Build history of the part. All positions in model axes, mm. A direction names the side the tool comes from. Coordinates: 2 decimals unless noted, no trailing zeros. Write each loop counter-clockwise with the first axis right and the second up, starting at its lowest first coordinate (ties: lowest second). Pieces come first, ordered by that corner, then holes.
from build123d import *

# Parameters (mm, degrees)
SKETCH1_R           = 4.5
SKETCH1_R_2         = 2.5
BOSS_EXTRUDE1_DEPTH = 3.6
SKETCH2_R           = 0.75
SKETCH2_R_2         = 6.25
SKETCH2_R_3         = 4.5
SKETCH2_R_4         = 2.5
SKETCH2_R_5         = 1.5
BOSS_EXTRUDE2_DEPTH = 2.7
SKETCH3_W           = 3
SKETCH3_H           = 0.5
SKETCH3_W_2         = 0.5
SKETCH3_H_2         = 3
BOSS_EXTRUDE3_DEPTH = 0.5


with BuildPart() as part:
    # Sketch1 → Boss-Extrude1 (new body)
    with BuildSketch(Plane(origin=(0, 0, 0), x_dir=(1, 0, 0), z_dir=(0, 1, 0))):
        with Locations(Location((0, 0, 0), (0, 0, 270))):
            Circle(SKETCH1_R)
        with Locations(Location((0, 0, 0), (0, 0, 270))):
            Circle(SKETCH1_R_2, mode=Mode.SUBTRACT)
    extrude(amount=BOSS_EXTRUDE1_DEPTH)

    # Sketch2 → Boss-Extrude2 (add)
    # profile 1 of 7: a face of its own
    with BuildSketch(Plane(origin=(0, 3.6, 0), x_dir=(1, 0, 0), z_dir=(0, 1, 0))):
        with BuildLine():
            ThreePointArc((4.419417382, -4.419417382), (0, -6.25), (-4.419417382, -4.419417382))
            Line((-4.419417382, -4.419417382), (-2, -16))
            ThreePointArc((-2, -16), (0, -18.265564437), (2, -16))
            Line((2, -16), (4.419417382, -4.419417382))
        make_face()
        with Locations(Location((0, -16.25, 0), (0, 0, 90))):
            Circle(SKETCH2_R, mode=Mode.SUBTRACT)
        with Locations(Location((0, -13.25, 0), (0, 0, 90))):
            Circle(SKETCH2_R, mode=Mode.SUBTRACT)
        with Locations(Location((0, -10.25, 0), (0, 0, 90))):
            Circle(SKETCH2_R, mode=Mode.SUBTRACT)
        with Locations(Location((0, -7.25, 0), (0, 0, 90))):
            Circle(SKETCH2_R, mode=Mode.SUBTRACT)
    # profile 2 of 7: a face of its own
    with BuildSketch(Plane(origin=(0, 3.6, 0), x_dir=(1, 0, 0), z_dir=(0, 1, 0))):
        with BuildLine():
            ThreePointArc((-4.419417382, -4.419417382), (-6.25, 0), (-4.419417382, 4.419417382))
            Line((-4.419417382, 4.419417382), (-16, 2))
            ThreePointArc((-16, 2), (-18.265564437, 0), (-16, -2))
            Line((-16, -2), (-4.419417382, -4.419417382))
        make_face()
        with Locations(Location((-16.25, 0, 0), (0, 0, 90))):
            Circle(SKETCH2_R, mode=Mode.SUBTRACT)
        with Locations(Location((-13.25, 0, 0), (0, 0, 90))):
            Circle(SKETCH2_R, mode=Mode.SUBTRACT)
        with Locations(Location((-10.25, 0, 0), (0, 0, 90))):
            Circle(SKETCH2_R, mode=Mode.SUBTRACT)
        with Locations(Location((-7.25, 0, 0), (0, 0, 90))):
            Circle(SKETCH2_R, mode=Mode.SUBTRACT)
    # profile 3 of 7: a face of its own
    with BuildSketch(Plane(origin=(0, 3.6, 0), x_dir=(1, 0, 0), z_dir=(0, 1, 0))):
        Circle(SKETCH2_R_2)
        with Locations(Location((0, 0, 0), (0, 0, 270))):
            Circle(SKETCH2_R_3, mode=Mode.SUBTRACT)
    # profile 4 of 7: a face of its own
    with BuildSketch(Plane(origin=(0, 3.6, 0), x_dir=(1, 0, 0), z_dir=(0, 1, 0))):
        with BuildLine():
            ThreePointArc((2, 16), (0, 18.265564437), (-2, 16))
            Line((-2, 16), (-4.419417382, 4.419417382))
            ThreePointArc((-4.419417382, 4.419417382), (0, 6.25), (4.419417382, 4.419417382))
            Line((4.419417382, 4.419417382), (2, 16))
        make_face()
        with Locations(Location((0, 7.25, 0), (0, 0, 90))):
            Circle(SKETCH2_R, mode=Mode.SUBTRACT)
        with Locations(Location((0, 10.25, 0), (0, 0, 90))):
            Circle(SKETCH2_R, mode=Mode.SUBTRACT)
        with Locations(Location((0, 13.25, 0), (0, 0, 90))):
            Circle(SKETCH2_R, mode=Mode.SUBTRACT)
        with Locations(Location((0, 16.25, 0), (0, 0, 90))):
            Circle(SKETCH2_R, mode=Mode.SUBTRACT)
    # profile 5 of 7: a face of its own
    with BuildSketch(Plane(origin=(0, 3.6, 0), x_dir=(1, 0, 0), z_dir=(0, 1, 0))):
        with BuildLine():
            Line((16, 2), (4.419417382, 4.419417382))
            ThreePointArc((4.419417382, 4.419417382), (5.774247078, 2.391771452), (6.25, 0))
            ThreePointArc((6.25, 0), (5.774247078, -2.391771452), (4.419417382, -4.419417382))
            Line((4.419417382, -4.419417382), (16, -2))
            ThreePointArc((16, -2), (18.265564437, 0), (16, 2))
        make_face()
        with Locations(Location((7.25, 0, 0), (0, 0, 90))):
            Circle(SKETCH2_R, mode=Mode.SUBTRACT)
        with Locations(Location((10.25, 0, 0), (0, 0, 90))):
            Circle(SKETCH2_R, mode=Mode.SUBTRACT)
        with Locations(Location((13.25, 0, 0), (0, 0, 90))):
            Circle(SKETCH2_R, mode=Mode.SUBTRACT)
        with Locations(Location((16.25, 0, 0), (0, 0, 90))):
            Circle(SKETCH2_R, mode=Mode.SUBTRACT)
    # profile 6 of 7: a face of its own
    with BuildSketch(Plane(origin=(0, 3.6, 0), x_dir=(1, 0, 0), z_dir=(0, 1, 0))):
        with Locations(Location((0, 0, 0), (0, 0, 270))):
            Circle(SKETCH2_R_3)
        with Locations(Location((0, 0, 0), (0, 0, 270))):
            Circle(SKETCH2_R_4, mode=Mode.SUBTRACT)
    # profile 7 of 7: a face of its own
    with BuildSketch(Plane(origin=(0, 3.6, 0), x_dir=(1, 0, 0), z_dir=(0, 1, 0))):
        with Locations(Location((0, 0, 0), (0, 0, 270))):
            Circle(SKETCH2_R_4)
        with Locations(Location((0, 0, 0), (0, 0, 90))):
            Circle(SKETCH2_R_5, mode=Mode.SUBTRACT)
    extrude(amount=BOSS_EXTRUDE2_DEPTH)

    # Sketch3 → Boss-Extrude3 (add)
    with BuildSketch(Plane.XZ.offset(-3.6)):
        with Locations((-6.336645362, -2.094924186)):
            Rectangle(SKETCH3_W, SKETCH3_H)
        with Locations((-2.456041922, -7.328306568)):
            Rectangle(SKETCH3_W_2, SKETCH3_H_2)
    extrude(amount=BOSS_EXTRUDE3_DEPTH)


solid = part.part
(1) Slice it at C-C, the plane x = 7.25. List the corners of the cut face in (y, z), and give its area (3 significant figures).
(2) Slice it at A-A, the plane y = 5. Give the number of separate pieces and of enclosed holes in the cut face, and give its area (3 significant figures).
(3) Two-plate mould, pull along Z, no slides. Class faces 3 (the cylindrical face through (17, 5, 0)), 4 (the flat face through (10.291, 4.931, -3.193)), 5 (the cylindrical face through (-18.265, 4.931, -0.048)): pulls with the +Z half, pulls with the -Z half, needs draft (parallel to the pull), parting line crosses it, or undercut.
(4) Probe L1, parallel to Z at x = -16.25, y = 5.3; L2, parallel to Y at x = -2, z = 15.5. List the from-to ranges inside material, lowest first.
(5) Slice it at D-D, the plane z = 3.5. List the corners of the cut face in (x, y).
(6) 3-axis set-ups, long thin cutter, end or side, ignore diameter. For faces 1 (the flat face through (-10.129, 4.931, -3.227)), 2 (the cylindrical face through (-2.44, 1.77, -0.54)): which of +Z, -Z, +X, -X, +Y, -Y reach the whole face in a straight line?
(7) Slice it at B-B, the plane z = -7.25. List the corners of the cut face in (x, y), and give its area (3 significant figures).
(8) Flat gauge pins, fed straight in: P1, Ø1, axis at x = -12, y = 3, coming from the +Z side; P2, Ø2, axis at x = 9.5, y = 5, coming from the +Z side; P3, Ø1.7, axis at x = 13.25, z = 0, coming from the -Y side; P4, Ø1, axis at y = 5.5, z = 8, coming from the -X side. Where does each tip first touch, or does it go through?
Results:
1. outline: (3.6, -3.83) - (6.3, -3.83) - (6.3, -0.75) - (3.6, -0.75) - close; (3.6, 0.75) - (6.3, 0.75) - (6.3, 3.83) - (3.6, 3.83) - close
1. area: 16.6 mm2
2. separate pieces: 1
2. enclosed holes: 17
2. area: 370 mm2
3. face 3: undercut
3. face 4: pulls with the -Z half
3. face 5: parting line crosses it
4. L1: z = -2.02 to -0.75, 0.75 to 2.02
4. L2: y = 3.6 to 6.3
5. outline: (-8.82, 3.6) - (-2.83, 3.6) - (-2.83, 0) - (2.83, 0) - (2.83, 3.6) - (8.82, 3.6) - (8.82, 6.3) - (-8.82, 6.3) - close
6. face 1: -Z, -X, +Y, -Y
6. face 2: -Y
7. outline: (-3.83, 3.6) - (-2.71, 3.6) - (-2.71, 3.1) - (-2.21, 3.1) - (-2.21, 3.6) - (-0.75, 3.6) - (-0.75, 6.3) - (-3.83, 6.3) - close; (0.75, 3.6) - (3.83, 3.6) - (3.83, 6.3) - (0.75, 6.3) - close
7. area: 16.9 mm2
8. P1: passes through
8. P2: stops at z = 3.57
8. P3: stops at y = 3.6
8. P4: stops at x = -3.78
